```python
from build123d import *

# Parameters (mm, degrees)
F0_W     = 76.2
F0_H     = 50.8
F0_R     = 12.7
F1_DEPTH = 12.7
F2_W     = 6.35
F2_H     = 50.8
F3_DEPTH = 2.54
F5_DEPTH = 50.801


with BuildPart() as f1:
    # F0 (on Top) → F1 (new body)
    with BuildSketch(Plane.XY):
        Rectangle(F0_W, F0_H)
        Circle(F0_R, mode=Mode.SUBTRACT)
    extrude(amount=F1_DEPTH)

    # F2 (on face) → F3 (cut)
    with BuildSketch(Plane.XY.offset(12.7)):
        with Locations((-32.385, 0)):
            Rectangle(F2_W, F2_H)
        with BuildLine():
            Line((-6.35, -10.9985226281), (-6.35, -25.4))
            Line((-6.35, -25.4), (6.35, -25.4))
            Line((6.35, -25.4), (6.35, -10.9985226281))
            ThreePointArc((6.35, -10.9985226281), (0, -12.7), (-6.35, -10.9985226281))
        make_face()
        with BuildLine():
            Line((6.35, 25.4), (-6.35, 25.4))
            Line((-6.35, 25.4), (-6.35, 10.9985226281))
            ThreePointArc((-6.35, 10.9985226281), (0, 12.7), (6.35, 10.9985226281))
            Line((6.35, 10.9985226281), (6.35, 25.4))
        make_face()
    extrude(amount=-F3_DEPTH, mode=Mode.SUBTRACT)

    # F4 (on face) → F5 (cut, through all)
    with BuildSketch(Plane.XZ.offset(25.4)):
        Polygon((28.0736974643, 12.7), (15.3736974643, 12.7), (12.4407580968, 7.62), (31.0066368318, 7.62), align=None)
    extrude(amount=-F5_DEPTH, mode=Mode.SUBTRACT)


solid = f1.part
```
Build history of the part. All positions in model axes, mm. A direction names the side the tool comes from. Round coordinates to 2 decimals unless told otherwise and drop trailing zeros. Write each loop counter-clockwise with the first axis right and the second up, starting at its lowest first coordinate (ties: lowest second). Pieces come first, ordered by that corner, then holes.
1) Band-saw the part on A-A, the plane x = 0. List the corners of the cut face in (y, z), and give its area (3 significant figures).
2) Drill centre lines: probe 1 along Y at (x, z) = (0, 7); probe 2 along X at (y, z) = (0, 3.75); probe 3 along X at (y, z) = (0, 9.25). Where is each one in solid material? Low to high.
3) 3-axis set-ups, long thin cutter, end or side, ignore diameter. For faces 1 (the flat face through (-29.21, 0, 11)), 2 (the flat face through (-37, 0, 12.7)), 3 (the flat face through (22, 0, 7.62)): which of +Z, -Z, +X, -X, +Y, -Y reach the whole face in a straight line?
4) Band-saw the part on B-B, the plane z = 4. List the corners of the cut face in (x, y).
5) Band-saw the part on D-D, the plane y = -19. List the corners of the cut face in (x, z).
6) Mould opens along X. For faces 4 (the flat face through (38.1, 0, 6)), 5 (the flat face through (29.561, -0.356, 10.124)), 6 (the flat face through (-38.1, 0, 6)), 7 (the flat face through (-18, 0, 12.7)) say: +X half, -X half, draft (parallel to the pull), parting line (faces both ways), or undercut.
7) Pin check, flat tips, straight feed: pin 1 (3 mm diameter, centred on x = -33, y = -7, fed in from +Z); pin 2 (1.5 mm diameter, centred on x = 18.5, y = 19, fed in from +Z). Stop position of each tip, or through.
8) Band-saw the part on C-C, the plane y = 0. List the corners of the cut face in (x, z), and give its area (3 significant figures).
Ans:
1. outline: (-25.4, 0) - (-12.7, 0) - (-12.7, 10.16) - (-25.4, 10.16) - close; (12.7, 0) - (25.4, 0) - (25.4, 10.16) - (12.7, 10.16) - close
1. area: 258 mm2
2. probe 1: y = -25.4 to -12.7, 12.7 to 25.4
2. probe 2: x = -38.1 to -12.7, 12.7 to 38.1
2. probe 3: x = -38.1 to -12.7, 12.7 to 13.38, 30.07 to 38.1
3. face 1: +Z, +Y, -Y
3. face 2: +Z, +X, -X, +Y, -Y
3. face 3: +Y, -Y
4. outline: (-38.1, -25.4) - (38.1, -25.4) - (38.1, 25.4) - (-38.1, 25.4) - close; hole circle Ø25.4 at (0, 0)
5. outline: (-38.1, 0) - (38.1, 0) - (38.1, 12.7) - (28.07, 12.7) - (31.01, 7.62) - (12.44, 7.62) - (15.37, 12.7) - (6.35, 12.7) - (6.35, 10.16) - (-6.35, 10.16) - (-6.35, 12.7) - (-29.21, 12.7) - (-29.21, 10.16) - (-35.56, 10.16) - (-35.56, 12.7) - (-38.1, 12.7) - close
6. face 4: +X half
6. face 5: undercut
6. face 6: -X half
6. face 7: draft
7. pin 1: stops at z = 10.16
7. pin 2: stops at z = 7.62
8. outline: (-38.1, 0) - (-12.7, 0) - (-12.7, 12.7) - (-29.21, 12.7) - (-29.21, 10.16) - (-35.56, 10.16) - (-35.56, 12.7) - (-38.1, 12.7) - close; (12.7, 0) - (38.1, 0) - (38.1, 12.7) - (28.07, 12.7) - (31.01, 7.62) - (12.7, 7.62) - close; (12.7, 8.07) - (15.37, 12.7) - (12.7, 12.7) - close
8. area: 550 mm2
